from build123d import *
from build123d.topology import SkipClean

# Parameters (mm, degrees)
ESQUISSE2_R             = 10
BOSS_EXTRU_1_DEPTH      = 48
ESQUISSE3_R             = 12.5
BOSS_EXTRU_2_DEPTH      = 81.25
CHANFREIN1_SIZE         = 1
ESQUISSE6_R             = 19
BOSS_EXTRU_3_DEPTH      = 60
BOSS_EXTRU_4_DEPTH      = 35
BOSS_EXTRU_4_DEPTH_BACK = 35
ESQUISSE7_W             = 38
ESQUISSE7_H             = 40.519603535
ENL_V_MAT_EXTRU_3_REACH = 207.478
BOSS_EXTRU_6_DEPTH      = 15
ESQUISSE16_W            = 38
ESQUISSE16_H            = 40
ENL_V_MAT_EXTRU_4_DEPTH = 20


with BuildPart() as part:
    # Esquisse2 → Boss.-Extru.1 (new body)
    with BuildSketch(Plane.XY):
        Circle(ESQUISSE2_R)
    extrude(amount=BOSS_EXTRU_1_DEPTH)

    # Esquisse3 → Boss.-Extru.2 (add)
    with BuildSketch(Plane.XY.offset(48)):
        Circle(ESQUISSE3_R)
    extrude(amount=BOSS_EXTRU_2_DEPTH)

    # Chanfrein1
    chanfrein1_edges = [part.edges().sort_by_distance(p)[0] for p in [
        (-10, 0, 0),
    ]]
    chamfer(chanfrein1_edges, length=CHANFREIN1_SIZE)

    # Esquisse6 → Boss.-Extru.3 (add)
    with BuildSketch(Plane.XY.offset(129.25)):
        Circle(ESQUISSE6_R)
    extrude(amount=BOSS_EXTRU_3_DEPTH)

    # Esquisse7 → Boss.-Extru.4 (add, two sides: drawn at the far end of the back side and taken through both)
    with BuildSketch(Plane(origin=(0, 0, 0), x_dir=(1, 0, 0), z_dir=(0, 1, 0)).offset(-BOSS_EXTRU_4_DEPTH_BACK)):
        with Locations((0, -171.990198233)):
            Rectangle(ESQUISSE7_W, ESQUISSE7_H)
    extrude(amount=BOSS_EXTRU_4_DEPTH + BOSS_EXTRU_4_DEPTH_BACK)

    # Esquisse12 → Enlèv. mat.-Extru.3 (cut, up to next)
    with BuildSketch(Plane(origin=(0, 35, 0), x_dir=(1, 0, 0), z_dir=(0, 1, 0)), mode=Mode.PRIVATE) as enl_v_mat_extru_3_sk1:
        with BuildLine():
            Line((-10.5, -192.25), (10.5, -192.25))
            ThreePointArc((10.5, -192.25), (0, -181.75), (-10.5, -192.25))
        make_face()
    enl_v_mat_extru_3_tool1 = extrude(enl_v_mat_extru_3_sk1.sketch, amount=-ENL_V_MAT_EXTRU_3_REACH, mode=Mode.PRIVATE) & part.part
    add(enl_v_mat_extru_3_tool1.solids().sort_by_distance((0, 35, 187.793662))[0], mode=Mode.SUBTRACT)

    # Esquisse15 → Boss.-Extru.6 (add)
    with BuildSketch(Plane(origin=(0, 35, 0), x_dir=(1, 0, 0), z_dir=(0, 1, 0))):
        with BuildLine():
            Line((-20, -192.25), (-10.5, -192.25))
            ThreePointArc((-10.5, -192.25), (0, -202.75), (10.5, -192.25))
            Line((10.5, -192.25), (20, -192.25))
            ThreePointArc((20, -192.25), (0, -212.25), (-20, -192.25))
        make_face()
    boss_extru_6 = extrude(amount=-BOSS_EXTRU_6_DEPTH)

    # Esquisse16 → Enlèv. mat.-Extru.4 (cut)
    with BuildSketch(Plane.XY.offset(192.25)):
        Rectangle(ESQUISSE16_W, ESQUISSE16_H)
    extrude(amount=-ENL_V_MAT_EXTRU_4_DEPTH, mode=Mode.SUBTRACT)

    # Symétrie2: Boss.-Extru.6 across plane
    with SkipClean():  # the faces are left unmerged after this step: merging them gives an invalid solid
        add(boss_extru_6.mirror(Plane.ZX))


solid = part.part
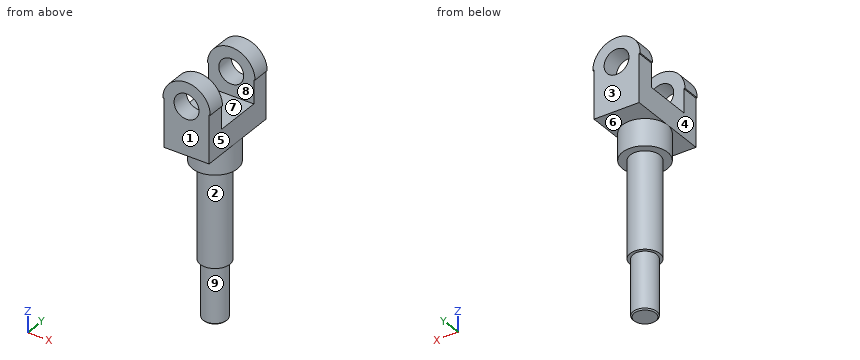
Could you check a few things on this model? Use its own coordinates, in mm. Face numbers are marked on the shaded views. A direction names the side the tool comes from. Round coordinates to 2 decimals unless told otherwise and drop trailing zeros. Order: outer loops, then holes, each group sorted by start corner. A loop starts at its lowest first (then second) coordinate and runs counter-clockwise, first axis right, second up.
(1) Which directions (+Z, -Z, +X, -X, +Y, -Y) give clear straight access to the entire face, cutting with the end or side of a thin tool? Please do the marked faces 1, 2, 3, 4 and 5.
Response values:
face 1: +Z, -Z, +X, -X, -Y
face 2: -Z
face 3: +Z, -Z, +X, -X, +Y
face 4: -Z, -X, +Y, -Y
face 5: -Z, +X, +Y, -Y
(2) Imagine slicing it at D-D (x = 17). Write out the boundary of the cut face in (y, z), plus the area to 3 significant figures.
Response values:
outline: (-35, 151.73) - (-8.49, 151.73) - (-8.49, 129.25) - (8.49, 129.25) - (8.49, 151.73) - (35, 151.73) - (35, 202.79) - (20, 202.79) - (20, 172.25) - (-20, 172.25) - (-20, 202.79) - (-35, 202.79) - close
area: 2,730 mm2
(3) If we mould it in two halves opening along Y, with no side actions, what happens to the marked faces 6, 7, 8 and 9? For each: released by +Y, released by -Y, zero draft, split by the parting line, or undercut.
Response values:
face 6: zero draft
face 7: undercut
face 8: undercut
face 9: split by the parting line
(4) Imagine slicing it at A-A (x = 0). Count the separate pieces of the cut face and the enclosed holes in it, plus the area to 3 significant figures.
Response values:
separate pieces: 3
enclosed holes: 0
area: 5,850 mm2
(5) Imagine slicing it at C-C (y = -27). Write out the boundary of the cut face in (x, z).
Response values:
outline: (-20, 192.25) - (-19, 192.25) - (-19, 151.73) - (19, 151.73) - (19, 192.25) - (20, 192.25) arc R20 ccw to start; hole circle Ø21 at (0, 192.25)
(6) I'm going to push flat-ended pins straight in: pin 1 (12 mm diameter, centred on x = -4, y = 2, fed in from +Z); pin 2 (0.8 mm diameter, centred on x = -19.5, y = 30, fed in from -Z); pin 3 (12 mm diameter, centred on y = 12.5, z = 174, fed in from -X); pin 4 (1 mm diameter, centred on x = -4, y = -7, fed in from -Z). Where does each tip first touch, or does it pass through?
Response values:
pin 1: stops at z = 172.25
pin 2: stops at z = 192.25
pin 3: stops at x = -19
pin 4: stops at z = 0
(7) Imagine slicing it at B-B (z = 176.5). Write out the boundary of the cut face in (x, y), plus the area to 3 significant figures.
Response values:
outline: (-19, -35) - (19, -35) - (19, -20) - (-19, -20) - close; (-19, 20) - (19, 20) - (19, 35) - (-19, 35) - close
area: 1,140 mm2
(8) Please list where these lines run through material, in increasing order: line 1 along Z through (x, y) = (0, 29); line 2 along Y through (x, z) = (11, 176.5); line 3 along X through (y, z) = (-25, 192).
Response values:
line 1: z = 151.73 to 181.75, 202.75 to 212.25
line 2: y = -35 to -20, 20 to 35
line 3: x = -19 to -10.5, 10.5 to 19
